```python
from build123d import *

# Parameters (mm, degrees)
SKETCH_1_R          = 19.5
EXTRUDE_1_DEPTH     = 32
SKETCH_2_R          = 7.88
EXTRUDE_2_DEPTH     = 5
CUT_EXTRUDE_1_REACH = 48.147
SKETCH_3_R          = 3
SKETCH_4_R          = 1.5
CUT_EXTRUDE_2_DEPTH = 10


with BuildPart() as part:
    # 草图1 → 凸台-拉伸1 (new body)
    with BuildSketch(Plane(origin=(0, 0, 0), x_dir=(0, 0, -1), z_dir=(1, 0, 0))):
        Circle(SKETCH_1_R)
    extrude(amount=EXTRUDE_1_DEPTH)

    # 草图2 → 凸台-拉伸2 (add)
    with BuildSketch(Plane(origin=(32, 0, 0), x_dir=(0, 0, -1), z_dir=(1, 0, 0))):
        Circle(SKETCH_2_R)
    extrude(amount=EXTRUDE_2_DEPTH)

    # 草图3 → 切除-拉伸1 (cut, up to next)
    with BuildSketch(Plane(origin=(37, 0, 0), x_dir=(0, 0, -1), z_dir=(1, 0, 0)), mode=Mode.PRIVATE) as cut_extrude_1_sk1:
        Circle(SKETCH_3_R)
    cut_extrude_1_tool1 = extrude(cut_extrude_1_sk1.sketch, amount=-CUT_EXTRUDE_1_REACH, mode=Mode.PRIVATE) & part.part
    add(cut_extrude_1_tool1.solids().sort_by_distance((37, 0, 0))[0], mode=Mode.SUBTRACT)

    # 草图4 → 切除-拉伸2 (cut)
    with BuildSketch(Plane(origin=(32, 0, 0), x_dir=(0, 0, -1), z_dir=(1, 0, 0))):
        with Locations((15, 0)):
            Circle(SKETCH_4_R)
        with Locations((-15, 0)):
            Circle(SKETCH_4_R)
    extrude(amount=-CUT_EXTRUDE_2_DEPTH, mode=Mode.SUBTRACT)


solid = part.part
```
Build history of the part. All positions in model axes, mm. A direction names the side the tool comes from. Round coordinates to 2 decimals unless told otherwise and drop trailing zeros. Order: outer loops, then holes, each group sorted by start corner. A loop starts at its lowest first (then second) coordinate and runs counter-clockwise, first axis right, second up. Notation, with made-up numbers: (58, 7.25) - (111, 7.25) arc R26 cw to (111, 42.25) - close; hole circle Ø4 at (-6, -29). An arc over 180 degrees is marked (long way). Use a Markdown table: item, result.
1) Saw through at A-A on z = 0. Write the cut outline in (x, y), and give its area (3 significant figures).
Recorded:
| item | result |
|---|---|
| outline | (0, -19.5) - (32, -19.5) - (32, -7.88) - (37, -7.88) - (37, -3) - (0, -3) - close; (0, 3) - (37, 3) - (37, 7.88) - (32, 7.88) - (32, 19.5) - (0, 19.5) - close |
| area | 1,100 mm² |
2) Tool access for faces 1 (the face through (0, -4, 0)), 2 (the face through (32, 0.3, -8.4)): list every direction of +Z, -Z, +X, -X, +Y, -Y with a clear straight run to the whole face (end or side of a thin tool).
Recorded:
| item | result |
|---|---|
| face 1 | +Z, -Z, -X, +Y, -Y |
| face 2 | +X |
3) Saw through at B-B on y = 0. Write the cut outline in (x, z), and give its area (3 significant figures).
Recorded:
| item | result |
|---|---|
| outline | (0, -19.5) - (32, -19.5) - (32, -16.5) - (22, -16.5) - (22, -13.5) - (32, -13.5) - (32, -7.88) - (37, -7.88) - (37, -3) - (0, -3) - close; (0, 3) - (37, 3) - (37, 7.88) - (32, 7.88) - (32, 13.5) - (22, 13.5) - (22, 16.5) - (32, 16.5) - (32, 19.5) - (0, 19.5) - close |
| area | 1,040 mm² |
4) Saw through at D-D on x = 12. Write the cut outline in (y, z), and give its area (3 significant figures).
Recorded:
| item | result |
|---|---|
| outline | circle Ø39 at (0, 0); hole circle Ø6 at (0, 0) |
| area | 1,170 mm² |
5) Flat gauge pins, fed straight in: pin 1 Ø8 at (x, z) = (23.5, 4) entering from +Y; pin 2 Ø1 at (x, y) = (12, -15) entering from +Z; pin 3 Ø10 at (x, z) = (31.5, -9.5) entering from +Y. Where does each tip first touch, or does it go through?
Recorded:
| item | result |
|---|---|
| pin 1 | stops at y = 19.5 |
| pin 2 | stops at z = 13.04 |
| pin 3 | stops at y = 18.97 |
6) Pull direction Y, two halves, no side cores. Call faces 3 (the face through (27.07, 0.07, -13.5)), 4 (the face through (37, 0.1, -3.4)), 5 (the face through (15.776, 19.334, 2.539)): pulls with the +Y half, pulls with the -Y half, needs draft (parallel to the pull), parting line crosses it, or undercut.
Recorded:
| item | result |
|---|---|
| face 3 | undercut |
| face 4 | needs draft |
| face 5 | parting line crosses it |
7) Wall check: L1, parallel to Y at x = 12, z = 0; L2, parallel to X at y = -3, z = 16; L3, parallel to Y at x = 30, z = -15. Give the ranges that are in metal, low to high.
Recorded:
| item | result |
|---|---|
| L1 | y = -19.5 to -3, 3 to 19.5 |
| L2 | x = 0 to 32 |
| L3 | y = -12.46 to -1.5, 1.5 to 12.46 |
8) Saw through at C-C on x = 30. Write the cut outline in (y, z).
Recorded:
| item | result |
|---|---|
| outline | circle Ø39 at (0, 0); hole circle Ø6 at (0, 0); hole circle Ø3 at (0, -15); hole circle Ø3 at (0, 15) |
